from build123d import *
from build123d.topology import SkipClean

# Parameters (mm, degrees)
SKETCH63_R                                           = 33.71
BOSS_EXTRUDE14_DEPTH                                 = 30
CUT_EXTRUDE16_START                                  = -1.56
CUT_EXTRUDE16_DEPTH                                  = 55.766975775
CUT_EXTRUDE17_DEPTH                                  = 57.326975775
CUT_EXTRUDE17_DEPTH_BACK                             = 57.326975775
BOSS_EXTRUDE15_DEPTH                                 = 12
CUT_EXTRUDE18_START                                  = -5.22
SKETCH69_R                                           = 2.1
CUT_EXTRUDE18_DEPTH                                  = 6
SKETCH70_R                                           = 3.36
SKETCH70_R_2                                         = 2.1
CUT_EXTRUDE19_DEPTH                                  = 63.259333256
CSK_FOR_M3_HEX_SOCKET_COUNTERSUNK_CAP_SC_D           = 3.6
CSK_FOR_M3_HEX_SOCKET_COUNTERSUNK_CAP_SC_DEPTH       = 14.440351168
CSK_FOR_M3_HEX_SOCKET_COUNTERSUNK_CAP_SC_CSINK_D     = 6.72
CSK_FOR_M3_HEX_SOCKET_COUNTERSUNK_CAP_SC_CSINK_ANGLE = 90
CSK_FOR_M3_HEX_SOCKET_COUNTERSUNK_CAP_SC_TIP         = 1.081549114
SKETCH74_R                                           = 44.614790837
CUT_EXTRUDE20_DEPTH                                  = 14
CSK_FOR_M6_HEX_SOCKET_COUNTERSUNK_CA_2_COUNT         = 2
CSK_FOR_M6_HEX_SOCKET_COUNTERSUNK_CA_2_PITCH         = 35.355339059
CSK_FOR_M6_HEX_SOCKET_COUNTERSUNK_CA_3_COUNT         = 2
CSK_FOR_M6_HEX_SOCKET_COUNTERSUNK_CA_3_PITCH         = 35.355339059
CSK_FOR_M6_HEX_SOCKET_COUNTERSUNK_CA_4_COUNT         = 2
CSK_FOR_M6_HEX_SOCKET_COUNTERSUNK_CA_4_PITCH         = 50
SKETCH79_R                                           = 6.72
CUT_EXTRUDE21_DEPTH                                  = 15


with BuildPart() as part:
    # Sketch63 → Boss-Extrude14 (new body)
    with BuildSketch(Plane(origin=(0, 0, 0), x_dir=(1, 0, 0), z_dir=(0, 1, 0))):
        with Locations(Location((0, 0, 0), (0, 0, 270))):
            Circle(SKETCH63_R)
    extrude(amount=BOSS_EXTRUDE14_DEPTH)

    # Sketch67 → Cut-Extrude16 (cut, through all)
    with BuildSketch(Plane.XY.offset(CUT_EXTRUDE16_START)):
        Polygon((-25.257756337, 0), (-19.816405169, 0), (-15.992682372, 8.2), (-29.081479134, 8.2), align=None)
        Polygon((19.742243663, 0), (25.183594831, 0), (29.007317628, 8.2), (15.918520866, 8.2), align=None)
    extrude(amount=-CUT_EXTRUDE16_DEPTH, mode=Mode.SUBTRACT)

    # Sketch67<3> → Cut-Extrude17 (cut, two sides: drawn at the far end of the back side and taken through both)
    with BuildSketch(Plane.XY.offset(-CUT_EXTRUDE17_DEPTH_BACK)):
        Polygon((-5.257756337, 0), (5.183594831, 0), (9.007317628, 8.2), (-9.081479134, 8.2), align=None)
    extrude(amount=CUT_EXTRUDE17_DEPTH + CUT_EXTRUDE17_DEPTH_BACK, mode=Mode.SUBTRACT)

    # Sketch68 → Boss-Extrude15 (add)
    with SkipClean():  # the faces are left unmerged after this step: merging them gives an invalid solid
        with BuildSketch(Plane.XZ):
            with BuildLine():
                Line((-5.257756337, 21.297448826), (-5.257756337, 33.297448826))
                ThreePointArc((-5.257756337, 33.297448826), (-12.10394362, 31.462019148), (-18.415011022, 28.235641821))
                Line((-18.415011022, 28.235641821), (-18.415011022, 21.297448826))
                Line((-18.415011022, 21.297448826), (-5.257756337, 21.297448826))
            make_face()
            with BuildLine():
                ThreePointArc((15.05537339, 30.161230613), (10.24115174, 32.116707662), (5.183594831, 33.309074509))
                Line((5.183594831, 33.309074509), (5.183594831, 21.297448826))
                Line((5.183594831, 21.297448826), (15.05537339, 21.297448826))
                Line((15.05537339, 21.297448826), (15.05537339, 30.161230613))
            make_face()
        extrude(amount=-BOSS_EXTRUDE15_DEPTH)

    # Sketch69 → Cut-Extrude18 (cut)
    with SkipClean():  # the faces are left unmerged after this step: merging them gives an invalid solid
        with BuildSketch(Plane(origin=(-0.037756337, 0, 0), x_dir=(0, 0, -1), z_dir=(1, 0, 0)).offset(CUT_EXTRUDE18_START)):
            with Locations((-28.297448826, 4.1)):
                Circle(SKETCH69_R)
        extrude(amount=-CUT_EXTRUDE18_DEPTH, mode=Mode.SUBTRACT)

    # Sketch70 → Cut-Extrude19 (cut, through all)
    # profile 1 of 2: a face of its own
    with SkipClean():  # the faces are left unmerged after this step: merging them gives an invalid solid
        with BuildSketch(Plane.ZY.offset(-9.183594831)):
            with Locations((28.297448826, 4.1)):
                Circle(SKETCH70_R)
            with Locations(Location((28.297448826, 4.1, 0), (0, 0, 180))):
                Circle(SKETCH70_R_2, mode=Mode.SUBTRACT)
        # profile 2 of 2: a face of its own
        with BuildSketch(Plane.ZY.offset(-9.183594831)):
            with Locations(Location((28.297448826, 4.1, 0), (0, 0, 180))):
                Circle(SKETCH70_R_2)
        extrude(amount=-CUT_EXTRUDE19_DEPTH, mode=Mode.SUBTRACT)

    # CSK for M3 Hex Socket Countersunk Cap Screw9
    with Locations(Plane(origin=(9.183594831, 0, 0), x_dir=(0, 0, -1), z_dir=(1, 0, 0))):
        with Locations((-28.297448826, 4.1)):
            CounterSinkHole(CSK_FOR_M3_HEX_SOCKET_COUNTERSUNK_CAP_SC_D / 2, CSK_FOR_M3_HEX_SOCKET_COUNTERSUNK_CAP_SC_CSINK_D / 2, depth=CSK_FOR_M3_HEX_SOCKET_COUNTERSUNK_CAP_SC_DEPTH, counter_sink_angle=CSK_FOR_M3_HEX_SOCKET_COUNTERSUNK_CAP_SC_CSINK_ANGLE)
            with Locations((0, 0, -(CSK_FOR_M3_HEX_SOCKET_COUNTERSUNK_CAP_SC_DEPTH + CSK_FOR_M3_HEX_SOCKET_COUNTERSUNK_CAP_SC_TIP / 2))):  # 118° drill point
                Cone(0, CSK_FOR_M3_HEX_SOCKET_COUNTERSUNK_CAP_SC_D / 2, CSK_FOR_M3_HEX_SOCKET_COUNTERSUNK_CAP_SC_TIP, mode=Mode.SUBTRACT)

    # Sketch74 → Cut-Extrude20 (cut)
    with SkipClean():  # the faces are left unmerged after this step: merging them gives an invalid solid
        with BuildSketch(Plane(origin=(0, 30, 0), x_dir=(1, 0, 0), z_dir=(0, 1, 0))):
            Circle(SKETCH74_R)
        extrude(amount=-CUT_EXTRUDE20_DEPTH, mode=Mode.SUBTRACT)

    # Sketch78 → CSK for M6 Hex Socket Countersunk Cap Screw4 (revolve, cut)
    with SkipClean():  # the faces are left unmerged after this step: merging them gives an invalid solid
        with BuildSketch(Plane(origin=(-17.67766953, 8.2, 17.67766953), x_dir=(0, 0, -1), z_dir=(1, 0, 0))):
            Polygon((0, 0), (0, 16.543012167), (3.5, 14.44), (3.5, 3.22), (6.72, 0), align=None)
        csk_for_m6_hex_socket_countersunk_cap_sc = revolve(axis=Axis((-17.67766953, 1.85, 17.67766953), (0, 1, 0)), mode=Mode.SUBTRACT)

    # CSK for M6 Hex Socket Countersunk Ca 2: CSK for M6 Hex Socket Countersunk Cap Screw4 ×2
    with SkipClean():  # the faces are left unmerged after this step: merging them gives an invalid solid
        with Locations(*[(i * CSK_FOR_M6_HEX_SOCKET_COUNTERSUNK_CA_2_PITCH, 0, 0) for i in range(1, CSK_FOR_M6_HEX_SOCKET_COUNTERSUNK_CA_2_COUNT)]):
            add(csk_for_m6_hex_socket_countersunk_cap_sc, mode=Mode.SUBTRACT)

    # CSK for M6 Hex Socket Countersunk Ca 3: CSK for M6 Hex Socket Countersunk Cap Screw4 ×2
    with SkipClean():  # the faces are left unmerged after this step: merging them gives an invalid solid
        with Locations(*[(0, 0, -i * CSK_FOR_M6_HEX_SOCKET_COUNTERSUNK_CA_3_PITCH) for i in range(1, CSK_FOR_M6_HEX_SOCKET_COUNTERSUNK_CA_3_COUNT)]):
            add(csk_for_m6_hex_socket_countersunk_cap_sc, mode=Mode.SUBTRACT)

    # CSK for M6 Hex Socket Countersunk Ca 4: CSK for M6 Hex Socket Countersunk Cap Screw4 ×2
    with SkipClean():  # the faces are left unmerged after this step: merging them gives an invalid solid
        with Locations(*[Vector(0.7071067811865438, 0, -0.7071067811865512) * (i * CSK_FOR_M6_HEX_SOCKET_COUNTERSUNK_CA_4_PITCH) for i in range(1, CSK_FOR_M6_HEX_SOCKET_COUNTERSUNK_CA_4_COUNT)]):
            add(csk_for_m6_hex_socket_countersunk_cap_sc, mode=Mode.SUBTRACT)

    # Sketch79 → Cut-Extrude21 (cut)
    with SkipClean():  # the faces are left unmerged after this step: merging them gives an invalid solid
        with BuildSketch(Plane.XZ.offset(-8.2)):
            with Locations((-17.67766953, -17.67766953)):
                Circle(SKETCH79_R)
            with Locations((17.67766953, -17.67766953)):
                Circle(SKETCH79_R)
            with Locations(Location((17.67766953, 17.67766953, 0), (0, 0, 90))):
                Circle(SKETCH79_R)
            with Locations(Location((-17.67766953, 17.67766953, 0), (0, 0, 90))):
                Circle(SKETCH79_R)
        extrude(amount=CUT_EXTRUDE21_DEPTH, mode=Mode.SUBTRACT)


solid = part.part
Could you check a few things on this model? Use its own coordinates, in mm. A direction names the side the tool comes from. Round coordinates to 2 decimals unless told otherwise and drop trailing zeros. Loops run counter-clockwise (first coordinate to the right, second up) from the corner with the lowest first, then second, coordinate; pieces in that order, holes last. Notation, with made-up numbers: (56.25, 42) - (107.25, 42) arc R18 ccw to (107.25, 65) - close; hole circle Ø9 at (60, 68.5). An arc over 180 degrees is marked (long way). Write item = value, one per line.
1) Imagine slicing it at D-D (x = 0). Please give me the cut outline in (y, z), and give its area (3 significant figures).
Computed:
outline = (8.2, -33.71) - (16, -33.71) - (16, 33.71) - (8.2, 33.71) - close
area = 526 mm2
2) I need wall thicknesses on line 1 along Z through (x, y) = (-17.5, 13.25); line 2 along X through (y, z) = (6.5, 18.5); line 3 along Z through (x, y) = (20, 9). Which ranges of each line are inside material? Lowest first, please. Write a range as from..to.
Computed:
line_1 = -28.81..-21.17, -14.18..14.18, 21.17..28.81
line_2 = -28.18..-24.35, -11.01..-8.29, 8.21..11.01, 24.35..28.18
line_3 = -27.14..-23.12, -12.23..12.23, 23.12..27.14
3) Imagine slicing it at C-C (x = 18.5). Give the number of separate pieces and of enclosed holes in the cut face, and give its area (3 significant figures).
Computed:
separate_pieces = 4
enclosed_holes = 0
area = 465 mm2
4) Imagine slicing it at A-A (z = 0). Please give me the cut outline in (x, y).
Computed:
outline = (-33.71, 0) - (-5.26, 0) - (-9.08, 8.2) - (9.01, 8.2) - (5.18, 0) - (33.71, 0) - (33.71, 16) - (-33.71, 16) - close
5) I'm going to push flat-ended pins straight in: P1, Ø8, axis at x = 17.68, z = -17.68, coming from the -Y side; P2, Ø4, axis at x = -21, y = 4, coming from the +Z side; P3, Ø10.5, axis at x = -22.5, z = -12, coming from the -Y side; P4, Ø12, axis at x = 17.68, z = -17.68, coming from the -Y side. Where does each tip first touch, or does it pass through?
Computed:
P1 = 10.92
P2 = 27.85
P3 = 0
P4 = 8.92
6) Imagine slicing it at B-B (y = 10). Please give me the cut outline in (x, z), and give its area (3 significant figures).
Computed:
outline = circle Ø67.42 at (0, 0); hole circle Ø9.84 at (-17.68, -17.68); hole circle Ø9.84 at (-17.68, 17.68); hole circle Ø9.84 at (17.68, -17.68); hole circle Ø9.84 at (17.68, 17.68)
area = 3,270 mm2
7) On a 3-axis mill with a long thin cutter (end or side, diameter ignored), from which of +Z, -Z, +X, -X, +Y, -Y can I reach the whole of each face in a straight line? I mean faces 4 (the flat face through (-11.258, 4, 28)), 5 (the flat face through (-5.258, 4, 26)), 6 (the flat face through (-6, 6, 21.297)). Say none if no direction works.
Computed:
face_4 = none
face_5 = +Z, -Z, -Y
face_6 = -Z
8) If we mould it in two halves opening along Z, with no side actions, what happens to faces 1 (the flat face through (-23, 5, -1.56)), 2 (the flat face through (0, 16, 0)), 3 (the cylindrical face through (10.96, 4.16, -17.5))? For each: pulls with the +Z half, pulls with the -Z half, needs draft (parallel to the pull), parting line crosses it, or undercut.
Computed:
face_1 = pulls with the -Z half
face_2 = needs draft
face_3 = undercut
